Autodesk Inventor part; units mm, degrees
ref_plane "YZ Plane" through (0, 0, 0) normal (1, 0, 0) x (0, 1, 0)
ref_plane "XZ Plane" through (0, 0, 0) normal (0, 1, 0) x (-1, 0, 0)
ref_plane "XY Plane" through (0, 0, 0) normal (0, 0, 1) x (1, 0, 0)
sketch "Sketch1" plane through (0, 0, 0) normal (0, 1, 0) x (-1, 0, 0)
  line L0 (-3, 1.2097) -> (3, 1.2097)
  line L1 (3, 1.2097) -> (3, -4.7903)
  line L2 (3, -4.7903) -> (-3, -4.7903)
  line L3 (-3, -4.7903) -> (-3, 1.2097)
  point P0 (0, 0)
  dimension "d0" = 6
  dimension "d1" = 6
extrude "Extrusion1" add sketch "Sketch1" along normal blind 8.7
sketch "Sketch2" plane through (0, 8.7, 0) normal (0, 1, 0) x (1, 0, 0)
  circle A0 centre (0, 1.7903) radius 3.5
  point P0 (0, 0)
  dimension "d4" = 7
extrude "Extrusion2" add sketch "Sketch2" along normal blind 8.4
sketch "Sketch3" plane through (0, 17.1, -1.7903) normal (0, 1, 0) x (1, 0, 0)
  circle A0 centre (0, 0) radius 3.5
  circle A1 centre (0, 0) radius 3.05
  point P0 (0, -1.7903)
  dimension "d7" = 6.1
extrude "Extrusion3" cut sketch "Sketch3" against normal blind 8 contours A1
sketch "Sketch4" plane through (-3, 0, -4.7903) normal (-1, 0, 0) x (0, 0, 1)
  circle A0 centre (3, 4) radius 3.24
  line L0 (6.5, 17.1) -> (-0.5, 17.1)
  point P0 (4.7903, 0)
  dimension "d10" = 6.48
  dimension "d11" = 13.1
extrude "Extrusion4" add sketch "Sketch4" along normal blind 12.7
chamfer "Chamfer1" distance 1 angle 45 5 edges at (3, 4.35, 1.2097) (3, 4.35, -4.7903) (3, 0, -1.7903) (0, 0, 1.2097) (0, 0, -4.7903)
properties part number "SMA_RightAngle"
Could you check a few things on this model? Use its own coordinates, in mm. A direction names the side the tool comes from. Give positions to 0.01 mm unless a question says otherwise; leave off trailing zeros. Order: outer loops, then holes, each group sorted by start corner. A loop starts at its lowest first (then second) coordinate and runs counter-clockwise, first axis right, second up. Notation, with made-up numbers: (0.5, 23.5) - (22.5, 23.5) arc R24 cw to (22.5, 36.5) - close; hole circle Ø11 at (84, 69). An arc over 180 degrees is marked (long way). One line per question, with ' | ' between items. Start each with the question number.
Item 1: I want a section at A-A on x = 0. Write out the boundary of the cut face in (y, z), then the cut area to 3 significant figures.
Item 2: Thinking about a two-plate mould opening in Z: for faces 6 (the flat face through (-1, 5, -4.79)), 7 (the flat face through (-0.53, 0.49, 0.7)), 8 (the cylindrical face through (-0.397, 13.156, -4.814)), which applies, pulls with the +Z half, pulls with the -Z half, needs draft (parallel to the pull), parting line crosses it, or undercut?
Item 3: I want a section at D-D on z = -0.5. Write out the boundary of the cut face in (x, y).
Item 4: I need wall thicknesses on probe 1 along Z at (x, y) = (0, 14.25); probe 2 along X at (y, z) = (5.5, -0.5); probe 3 along Z at (x, y) = (-2.75, 5). Which ranges of each line are inside material? Lowest first, please. Write a range as [from, to].
Item 5: I'm going to push flat-ended pins straight in: pin 1 Ø1.3 at (x, z) = (-2.5, -4.5) entering from +Y; pin 2 Ø3 at (y, z) = (8.5, -3.5) entering from +X; pin 3 Ø3 at (x, z) = (0, -2) entering from +Y; pin 4 Ø8 at (x, y) = (-9.5, 10) entering from -Z. Where does each tip first touch, or does it pass through?
Item 6: I want a section at C-C on z = -3. Write out the boundary of the cut face in (x, y), then the cut area to 3 significant figures.
Item 7: For faces 1 (the flat face through (0, 9.1, -2)), 2 (the flat face through (-3, 0.4, -1.7)), 3 (the cylindrical face through (-9.261, 7.163, -2.493)), 4 (the flat face through (-2.7, 8.7, -4.4)), 5 (the flat face through (0, 5, 1.21)), which set-ups out of +Z, -Z, +X, -X, +Y, -Y let a thin tool reach every point of the face, with its end or its side?
Item 8: I want a section at B-B on y = 4. Write out the boundary of the cut face in (x, z).
Verdict:
1) outline: (0, -3.79) - (1, -4.79) - (8.7, -4.79) - (8.7, -5.29) - (17.1, -5.29) - (17.1, -4.84) - (9.1, -4.84) - (9.1, 1.26) - (17.1, 1.26) - (17.1, 1.71) - (8.7, 1.71) - (8.7, 1.21) - (1, 1.21) - (0, 0.21) - close | area: 61.2 mm^2
2) face 6: pulls with the -Z half | face 7: pulls with the +Z half | face 8: undercut
3) outline: (-15.7, 1.03) - (-3, 1.03) - (-3, 0) - (2, 0) - (3, 1) - (3, 8.7) - (3.25, 8.7) - (3.25, 17.1) - (2.76, 17.1) - (2.76, 9.1) - (-2.76, 9.1) - (-2.76, 17.1) - (-3.25, 17.1) - (-3.25, 8.7) - (-3, 8.7) - (-3, 6.97) - (-15.7, 6.97) - close
4) probe 1: [-5.29, -4.84], [1.26, 1.71] | probe 2: [-15.7, 3] | probe 3: [-4.79, 1.21]
5) pin 1: y = 17.1 | pin 2: x = 3.49 | pin 3: y = 9.1 | pin 4: z = -4.34
6) outline: (-15.7, 0.99) - (-3, 0.99) - (-3, 0) - (2, 0) - (3, 1) - (3, 8.7) - (3.28, 8.7) - (3.28, 17.1) - (2.8, 17.1) - (2.8, 9.1) - (-2.8, 9.1) - (-2.8, 17.1) - (-3.28, 17.1) - (-3.28, 8.7) - (-3, 8.7) - (-3, 7.01) - (-15.7, 7.01) - close | area: 138 mm^2
7) face 1: +Y | face 2: -X, -Y | face 3: -X | face 4: -Z, -X, +Y | face 5: +Z, +X, -Y
8) outline: (-15.7, -5.03) - (-3, -5.03) - (-3, -4.79) - (2, -4.79) - (3, -3.79) - (3, 0.21) - (2, 1.21) - (-3, 1.21) - (-3, 1.45) - (-15.7, 1.45) - close
